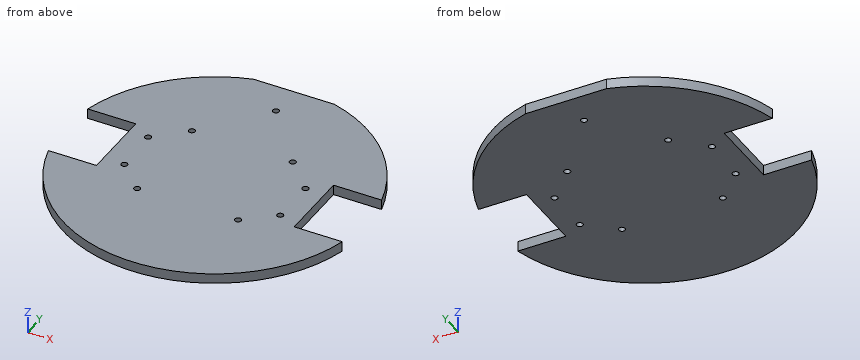
```python
from build123d import *

# Parameters (mm, degrees)
F0_R      = 75
F1_DEPTH  = 5
F2_W      = 26
F2_H      = 36
F3_DEPTH  = 25
F4_W      = 26
F4_H      = 36
F5_DEPTH  = 25
F6_W      = 40
F6_H      = 5.71822
F7_DEPTH  = 25
F8_R      = 1.55
F9_DEPTH  = 25
F10_R     = 1.55
F11_DEPTH = 25
F12_R     = 1.55
F13_DEPTH = 25
F14_R     = 1.55
F15_DEPTH = 25


with BuildPart() as f1:
    # F0 (on Top) → F1 (new body)
    with BuildSketch(Plane.XY):
        Circle(F0_R)
    extrude(amount=F1_DEPTH)

    # F2 (on Top) → F3 (cut)
    with BuildSketch(Plane.XY):
        with Locations((62, 0)):
            Rectangle(F2_W, F2_H)
    extrude(amount=F3_DEPTH, mode=Mode.SUBTRACT)

    # F4 (on Top) → F5 (cut)
    with BuildSketch(Plane.XY):
        with Locations((-62, 0)):
            Rectangle(F4_W, F4_H)
    extrude(amount=F5_DEPTH, mode=Mode.SUBTRACT)

    # F6 (on Top) → F7 (cut)
    with BuildSketch(Plane.XY):
        with Locations((0, 75.143271)):
            Rectangle(F6_W, F6_H)
    extrude(amount=F7_DEPTH, mode=Mode.SUBTRACT)

    # F8 (on face) → F9 (cut)
    with BuildSketch(Plane.XY.offset(5)):
        with Locations((-25, -25)):
            Circle(F8_R)
        with Locations((-25, 25)):
            Circle(F8_R)
        with Locations((25, 25)):
            Circle(F8_R)
        with Locations((25, -25)):
            Circle(F8_R)
    extrude(amount=-F9_DEPTH, mode=Mode.SUBTRACT)

    # F10 (on face) → F11 (cut)
    with BuildSketch(Plane.XY.offset(5)):
        with Locations((39.45, 9.95)):
            Circle(F10_R)
        with Locations((39.45, -13.15)):
            Circle(F10_R)
    extrude(amount=-F11_DEPTH, mode=Mode.SUBTRACT)

    # F12 (on face) → F13 (cut)
    with BuildSketch(Plane.XY.offset(5)):
        with Locations((-39.45, 11.638757)):
            Circle(F12_R)
        with Locations((-38.729364, -11.45)):
            Circle(F12_R)
    extrude(amount=-F13_DEPTH, mode=Mode.SUBTRACT)

    # F14 (on face) → F15 (cut)
    with BuildSketch(Plane.XY.offset(5)):
        with Locations((0, 55.734161)):
            Circle(F14_R)
    extrude(amount=-F15_DEPTH, mode=Mode.SUBTRACT)


solid = f1.part
```
Source: CAD feature listing. Evaluate the final solid. Frame: model axes, mm. Round coordinates to 2 decimals unless told otherwise and drop trailing zeros. Write each loop counter-clockwise with the first axis right and the second up, starting at its lowest first coordinate (ties: lowest second). Pieces come first, ordered by that corner, then holes. Notation, with made-up numbers: M 49.5,-29.75 L 79.5,-29.75 A21 cw 79.5,6.25 Z; hole C 66,44 d10. An arc over 180 degrees is marked long. Answer as a JSON object with one key per item and string values. Group by question number.
(1) Section query A-A on z = 0.85. State how many separate pieces and enclosed holes the cut face has, then the cut area to 3 significant figures.
(2) Section query B-B on y = 5.5. Output: boundary loops of the cut face in (x, z), then the cut area to 3 significant figures.
(3) First-contact query: pin 1 (1.9 mm diameter, centred on x = 0, y = 55.73, fed in from +Z); pin 2 (2.5 mm diameter, centred on y = 5.5, z = 2.5, fed in from -X); pin 3 (2.5 mm diameter, centred on x = 66.5, z = 2.5, fed in from +Y); pin 4 (1.5 mm diameter, centred on y = -0.5, z = 2, fed in from +X). Flat tips, straight axial feed; report the tip coordinate or a pass-through.
(4) Ray query, line 1 (Y direction, x = -25, z = 2.95); line 2 (Y direction, x = -40, z = 3.25); line 3 (X direction, y = -11.5, z = 3.95). Return the intervals inside material, ascending. Write a range as [from, to].
(5) Section query C-C on x = 47. Output: boundary loops of the cut face in (y, z).
Computed values:
{
 "1": {"separate pieces": "1", "enclosed holes": "9", "area": "15,700 mm^2"},
 "2": {"outline": "M -49,0 L 49,0 L 49,5 L -49,5 Z", "area": "490 mm^2"},
 "3": {"pin 1": "through", "pin 2": "x = -49", "pin 3": "y = 36.98", "pin 4": "x = 49"},
 "4": {"line 1": "[-70.71, -26.55], [-23.45, 23.45], [26.55, 70.71]", "line 2": "[-63.44, -12.34], [-10.56, 10.19], [13.09, 63.44]", "line 3": "[-49, -40.28], [-37.18, 49]"},
 "5": {"outline": "M -58.45,0 L 58.45,0 L 58.45,5 L -58.45,5 Z"}
}
